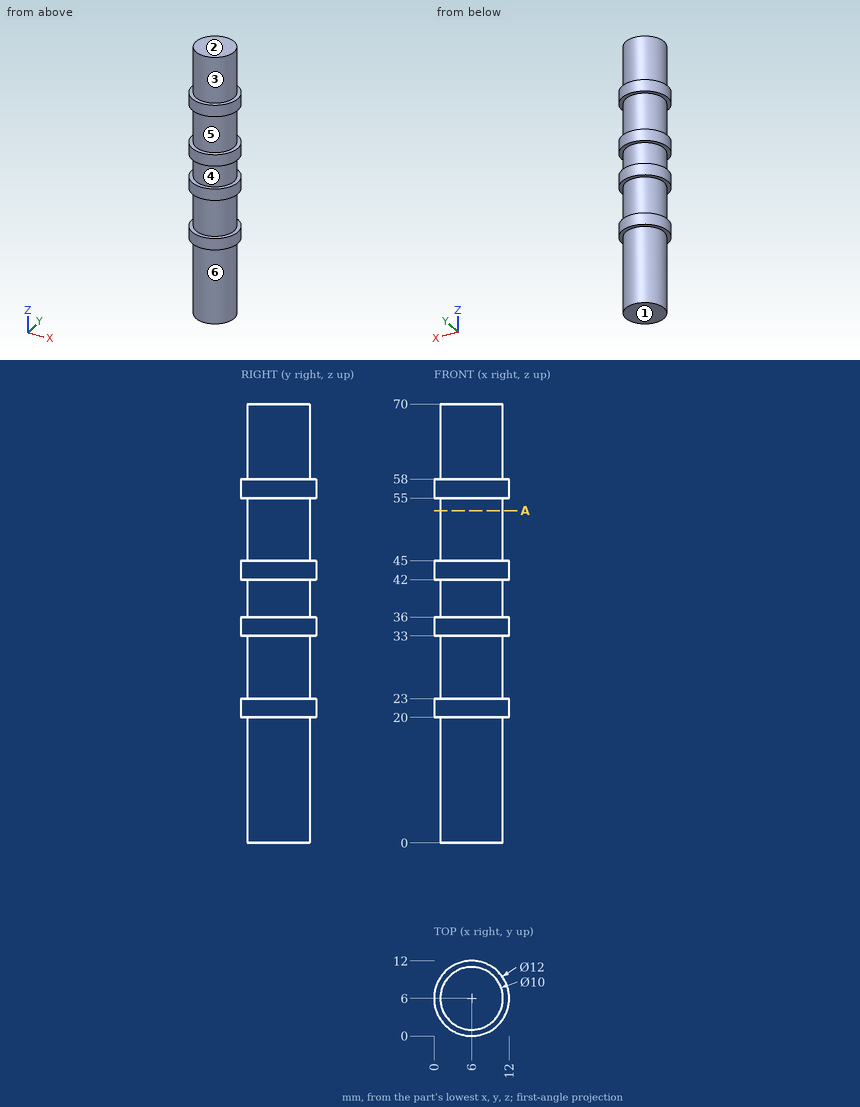
Design review of the part shown in the three views and the two pictorial views. Dimensions are in mm from the part's minimum x, y and z. A direction names the side the tool comes from. Coordinates: 2 decimals unless noted, no trailing zeros. Write each loop counter-clockwise with the first axis right and the second up, starting at its lowest first coordinate (ties: lowest second). Pieces come first, ordered by that corner, then holes.
(1) Add section A-A on z = 53. Give the boundary of the cut face in (x, y).
(2) Tool access review of the marked faces 5 and 6: name each direction out of +Z, -Z, +X, -X, +Y, -Y from which nothing blocks a thin tool from reaching the whole face with its end or side.
(3) For pin 1 Ø5 at (x, z) = (10.5, 54) entering from +Y, flat-tipped, find the tip position at first contact; note if it passes through.
(4) The part is to be moulded in two halves that separate along Z. For the marked faces 1, 2, 3 and 4, say which applies: +Z half, -Z half, draft (parallel to the pull), parting line (faces both ways), or undercut.
(5) Wall thickness on probe 1 along Z at (x, y) = (0.5, 6.5); probe 2 along X at (y, z) = (5.5, 54); probe 3 along Y at (x, z) = (3.25, 48): over which ranges is each line inside the solid? List them lowest first.
Answer sheet:
1. outline: circle Ø10 at (6, 6)
2. face 5: none
2. face 6: -Z
3. pin 1: stops at y = 11.58
4. face 1: -Z half
4. face 2: +Z half
4. face 3: draft
4. face 4: undercut
5. probe 1: z = 20 to 23, 33 to 36, 42 to 45, 55 to 58
5. probe 2: x = 1.03 to 10.97
5. probe 3: y = 1.82 to 10.18
